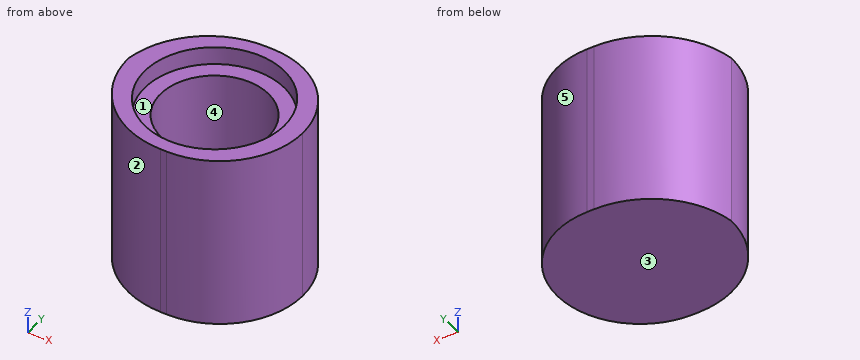
```python
from build123d import *

# Parameters (mm, degrees)
SKETCH1_W                = 39
SKETCH1_H                = 7.38
BOSS_EXTRUDE1_DEPTH      = 7.76
SKETCH2_R                = 2.4
CUT_EXTRUDE1_DEPTH       = 7.76
CUT_EXTRUDE2_OUTLINE_R   = 3.1
CUT_EXTRUDE2_OUTLINE_R_2 = 2.4
CUT_EXTRUDE2_DEPTH       = 0.8
CUT_EXTRUDE3_START       = 6.96
CUT_EXTRUDE3_OUTLINE_R   = 3.1
CUT_EXTRUDE3_OUTLINE_R_2 = 2.4
CUT_EXTRUDE3_DEPTH       = 0.8
LPATTERN3_COUNT          = 3
LPATTERN3_PITCH          = 7.79
LPATTERN6_COUNT          = 3
LPATTERN6_PITCH          = 7.79
FILLET1_R                = 3.69
FILLET2_R                = 3.69
FILLET3_R                = 3.69
FILLET4_R                = 3.69
SKETCH4_W                = 32.047846992
SKETCH4_H                = 7.400170021
CUT_EXTRUDE4_DEPTH       = 10
FILLET6_R                = 4
FILLET7_R                = 4
BOSS_EXTRUDE2_START      = -0.8
BOSS_EXTRUDE2_OUTLINE_R  = 3.1
BOSS_EXTRUDE2_DEPTH      = 0.8


with BuildPart() as part:
    # Sketch1 → Boss-Extrude1 (new body)
    with BuildSketch(Plane.XY):
        with Locations((19.5, 3.69)):
            Rectangle(SKETCH1_W, SKETCH1_H)
    extrude(amount=BOSS_EXTRUDE1_DEPTH)

    # Sketch2 → Cut-Extrude1 (cut)
    with BuildSketch(Plane.XY.offset(7.76)):
        with Locations((19.5, 3.69)):
            Circle(SKETCH2_R)
    cut_extrude1 = extrude(amount=-CUT_EXTRUDE1_DEPTH, mode=Mode.SUBTRACT)

    # Cut-Extrude2: read off the stored shape, not the designer's step
    # Cut-Extrude2 outline → Cut-Extrude2 (cut)
    with BuildSketch(Plane.XY):
        with Locations((19.5, 3.69)):
            Circle(CUT_EXTRUDE2_OUTLINE_R)
        with Locations((19.5, 3.69)):
            Circle(CUT_EXTRUDE2_OUTLINE_R_2, mode=Mode.SUBTRACT)
    cut_extrude2 = extrude(amount=CUT_EXTRUDE2_DEPTH, mode=Mode.SUBTRACT)

    # Cut-Extrude3: read off the stored shape, not the designer's step
    # Cut-Extrude3 outline → Cut-Extrude3 (cut)
    with BuildSketch(Plane.XY.offset(CUT_EXTRUDE3_START)):
        with Locations((19.5, 3.69)):
            Circle(CUT_EXTRUDE3_OUTLINE_R)
        with Locations((19.5, 3.69)):
            Circle(CUT_EXTRUDE3_OUTLINE_R_2, mode=Mode.SUBTRACT)
    cut_extrude3 = extrude(amount=CUT_EXTRUDE3_DEPTH, mode=Mode.SUBTRACT)

    # LPattern3: Cut-Extrude1, Cut-Extrude2, Cut-Extrude3 ×3
    with Locations(*[(-i * LPATTERN3_PITCH, 0, 0) for i in range(1, LPATTERN3_COUNT)]):
        add(cut_extrude1, mode=Mode.SUBTRACT)
        add(cut_extrude2, mode=Mode.SUBTRACT)
        add(cut_extrude3, mode=Mode.SUBTRACT)

    # LPattern6: Cut-Extrude1, Cut-Extrude2, Cut-Extrude3 ×3
    with Locations(*[(i * LPATTERN6_PITCH, 0, 0) for i in range(1, LPATTERN6_COUNT)]):
        add(cut_extrude1, mode=Mode.SUBTRACT)
        add(cut_extrude2, mode=Mode.SUBTRACT)
        add(cut_extrude3, mode=Mode.SUBTRACT)

    # Fillet1
    fillet1_edges = [part.edges().sort_by_distance(p)[0] for p in [
        (0, 7.38, 3.88),
    ]]
    fillet(fillet1_edges, radius=FILLET1_R)

    # Fillet2
    fillet2_edges = [part.edges().sort_by_distance(p)[0] for p in [
        (0, 0, 3.88),
    ]]
    fillet(fillet2_edges, radius=FILLET2_R - 0.0001)  # a hair under: the kernel refuses the full size

    # Fillet3
    fillet3_edges = [part.edges().sort_by_distance(p)[0] for p in [
        (39, 7.38, 3.88),
    ]]
    fillet(fillet3_edges, radius=FILLET3_R)

    # Fillet4
    fillet4_edges = [part.edges().sort_by_distance(p)[0] for p in [
        (39, 0, 3.88),
    ]]
    fillet(fillet4_edges, radius=FILLET4_R - 0.0001)  # a hair under: the kernel refuses the full size

    # Sketch4 → Cut-Extrude4 (cut)
    with BuildSketch(Plane(origin=(0, 0, 0), x_dir=(-1, 0, 0), z_dir=(0, 0, -1))):
        with Locations((-15.027741002, 3.700085011)):
            Rectangle(SKETCH4_W, SKETCH4_H)
    extrude(amount=-CUT_EXTRUDE4_DEPTH, mode=Mode.SUBTRACT)

    # Fillet6
    fillet6_edges = [part.edges().sort_by_distance(p)[0] for p in [
        (31.051664498, 0, 3.88),
    ]]
    fillet(fillet6_edges, radius=FILLET6_R)

    # Fillet7
    # the kernel refuses this fillet: 4 mm, written as the material it takes off along each edge
    with BuildSketch(Plane(origin=(31.051664498, 7.38, -9.8791447), x_dir=(0, -1, 0), z_dir=(0, 0, 1))) as fillet7_piece_1:
        with BuildLine():
            CenterArc((4, 3.95165788), FILLET7_R, 180, 81.083203747)
            Line((0, 3.95165788), (-0.08, 3.95165788))
            Line((-0.08, 3.95165788), (-0.08, 0))
            Line((-0.08, 0), (0, -0.08))
            ThreePointArc((0, -0.08), (1.69, -0.08), (3.3676, -0.079033158))
            Line((3.3676, -0.079033158), (3.38, 0))
        make_face()
    extrude(amount=27.5182894, mode=Mode.SUBTRACT)

    # Boss-Extrude2: read off the stored shape, not the designer's step
    # Boss-Extrude2 outline → Boss-Extrude2 (add)
    with BuildSketch(Plane(origin=(0, 0, 0), x_dir=(-1, 0, 0), z_dir=(0, 0, -1)).offset(BOSS_EXTRUDE2_START)):
        with Locations((-35.08, 3.69)):
            Circle(BOSS_EXTRUDE2_OUTLINE_R)
    extrude(amount=BOSS_EXTRUDE2_DEPTH)


solid = part.part
```
Could you check a few things on this model? Use its own coordinates, in mm. Face numbers are marked on the shaded views. A direction names the side the tool comes from. Round coordinates to 2 decimals unless told otherwise and drop trailing zeros. Write each loop counter-clockwise with the first axis right and the second up, starting at its lowest first coordinate (ties: lowest second). Pieces come first, ordered by that corner, then holes.
(1) If I drill on probe 1 along Y at (x, z) = (35.08, 5.25); probe 2 along Y at (x, z) = (35.08, 7.35); probe 3 along Z at (x, y) = (32.5, 3.5), over which ranges is the centre line in solid material (lowest first)?
Findings below:
probe 1: y = 0 to 1.29, 6.09 to 7.38
probe 2: y = 0 to 0.59, 6.79 to 7.38
probe 3: z = 0 to 6.96
(2) Suppose I cut it at B-B on y = 3.25. Write out the boundary of the cut face in (x, z), and give its area (3 significant figures).
Findings below:
outline: (31.12, 0) - (38.97, 0) - (38.97, 7.76) - (38.15, 7.76) - (38.15, 6.96) - (37.44, 6.96) - (37.44, 0.8) - (32.72, 0.8) - (32.72, 6.96) - (32.01, 6.96) - (32.01, 7.76) - (31.12, 7.76) - close
area: 26.9 mm2
(3) Suppose I cut it at D-D on y = 6.25. Write out the boundary of the cut face in (x, z), and give its area (3 significant figures).
Findings below:
outline: (32.22, 0) - (37.97, 0) - (37.97, 7.76) - (36.83, 7.76) - (36.83, 6.96) - (33.33, 6.96) - (33.33, 7.76) - (32.22, 7.76) - close
area: 41.8 mm2
(4) Suppose I cut it at C-C on x = 34.25. Write out the boundary of the cut face in (y, z), and give its area (3 significant figures).
Findings below:
outline: (0.08, 0) - (7.31, 0) - (7.31, 7.76) - (6.68, 7.76) - (6.68, 6.96) - (5.94, 6.96) - (5.94, 0.8) - (1.44, 0.8) - (1.44, 6.96) - (0.7, 6.96) - (0.7, 7.76) - (0.08, 7.76) - close
area: 23.6 mm2
(5) Which directions (+Z, -Z, +X, -X, +Y, -Y) give clear straight access to the entire face, cutting with the end or side of a thin tool? Please do the marked faces 1 and 2.
Findings below:
face 1: +Z
face 2: +Z, -Z, -X, -Y
(6) Thinking about a two-plate mould opening in Y: for the marked faces 3, 4 and 5, which applies, +Y half, -Y half, draft (parallel to the pull), parting line (faces both ways), or undercut?
Findings below:
face 3: draft
face 4: undercut
face 5: +Y half
(7) For pin 1 (3 mm diameter, centred on x = 32, y = 5.5, fed in from -Z); pin 2 (1.9 mm diameter, centred on x = 33.5, y = 2.5, fed in from +Z); pin 3 (3 mm diameter, centred on y = 6.5, z = 4.5, fed in from -X), each with a flat end and sliding along its axis, tell me the tip position at first contact or that it passes through.
Findings below:
pin 1: stops at z = 0
pin 2: stops at z = 6.96
pin 3: stops at x = 31.35
